Input: part model. Units: mm. Frame: model coordinates. Face numbers are marked on the shaded views. Give positions to 0.01 mm unless a question says otherwise; leave off trailing zeros. Order: outer loops, then holes, each group sorted by start corner. A loop starts at its lowest first (then second) coordinate and runs counter-clockwise, first axis right, second up. Notation, with made-up numbers: (-12.5, 15) - (46.5, 15) arc R15 cw to (46.5, 38) - close; hole circle Ø8 at (-9, 82). An arc over 180 degrees is marked (long way). Use a Markdown table: item, result.
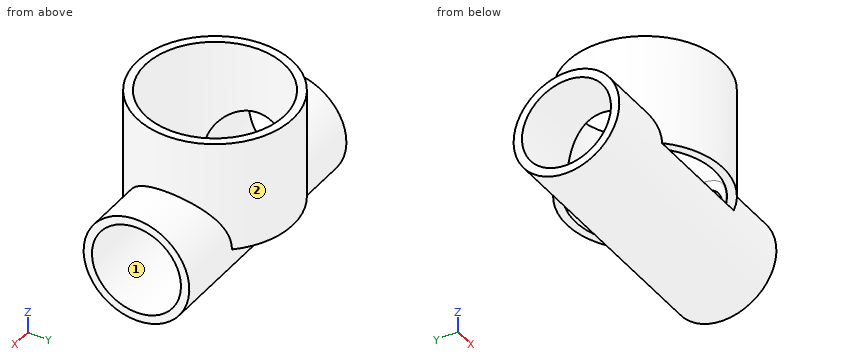
from build123d import *

# Parameters (mm, degrees)
SKETCH_1_R               = 14
SKETCH_1_R_2             = 12.5
EXTRUDE_1_DEPTH          = 20
EXTRUDE_2_DEPTH          = 22.5
EXTRUDE_2_DEPTH_BACK     = 22.5
SKETCH_2_R               = 9.5
SKETCH_2_R_2             = 8
CUT_EXTRUDE_1_DEPTH      = 40.654760284
CUT_EXTRUDE_1_DEPTH_BACK = 20
SKETCH_3_R               = 12.5
CUT_EXTRUDE_2_DEPTH      = 52.195703099
CUT_EXTRUDE_2_DEPTH_BACK = 52.195703099
SKETCH_4_R               = 8


with BuildPart() as part:
    # Sketch 1 → Extrude 1 (new body)
    with BuildSketch(Plane.XY):
        Circle(SKETCH_1_R)
        Circle(SKETCH_1_R_2, mode=Mode.SUBTRACT)
    extrude(amount=EXTRUDE_1_DEPTH)

    # Sketch 2 → Extrude 2 (add, two sides: drawn at the far end of the back side and taken through both)
    with BuildSketch(Plane(origin=(0, 0, 0), x_dir=(0, 0, -1), z_dir=(1, 0, 0)).offset(-EXTRUDE_2_DEPTH_BACK)):
        Circle(SKETCH_2_R)
        Circle(SKETCH_2_R_2, mode=Mode.SUBTRACT)
    extrude(amount=EXTRUDE_2_DEPTH + EXTRUDE_2_DEPTH_BACK)

    # Sketch 3 → Cut-Extrude 1 (cut, two sides: drawn at the far end of the back side and taken through both)
    with BuildSketch(Plane.XY.offset(20).offset(-CUT_EXTRUDE_1_DEPTH_BACK)):
        with Locations(Location((0, 0, 0), (0, 0, 219.7918195))):
            Circle(SKETCH_3_R)
    extrude(amount=CUT_EXTRUDE_1_DEPTH + CUT_EXTRUDE_1_DEPTH_BACK, mode=Mode.SUBTRACT)

    # Sketch 4 → Cut-Extrude 2 (cut, two sides: drawn at the far end of the back side and taken through both)
    with BuildSketch(Plane(origin=(22.5, 0, 0), x_dir=(0, 0, -1), z_dir=(1, 0, 0)).offset(-CUT_EXTRUDE_2_DEPTH_BACK)):
        Circle(SKETCH_4_R)
    extrude(amount=CUT_EXTRUDE_2_DEPTH + CUT_EXTRUDE_2_DEPTH_BACK, mode=Mode.SUBTRACT)


solid = part.part
1. Section query D-D (z = 8.75). Return loops of the section in (x, y).
Response:
| item | result |
|---|---|
| outline | (-22.5, -3.7) - (-13.5, -3.7) arc R14 ccw to (13.5, -3.7) - (22.5, -3.7) - (22.5, 3.7) - (13.5, 3.7) arc R14 ccw to (-13.5, 3.7) - (-22.5, 3.7) - close; hole circle Ø25 at (0, 0) |
2. Pin query (flat end, axial travel): pin 1 (3 mm diameter, centred on x = -7.5, z = 14, fed in from +Y); pin 2 (5 mm diameter, centred on x = 4.5, y = 12.5, fed in from -Z); pin 3 (1.7 mm diameter, centred on x = 4, y = 9, fed in from +Z). Return the tip coordinate at first contact, or that it passes through.
Response:
| item | result |
|---|---|
| pin 1 | stops at y = 12.65 |
| pin 2 | stops at z = 0 |
| pin 3 | stops at z = 0 |
3. Section query C-C (z = -6). Return loops of the section in (x, y).
Response:
| item | result |
|---|---|
| outline | (-22.5, -7.37) - (22.5, -7.37) - (22.5, -5.29) - (-22.5, -5.29) - close; (-22.5, 5.29) - (22.5, 5.29) - (22.5, 7.37) - (-22.5, 7.37) - close |
4. Material intervals for line 1 along X through (y, z) = (0, 15.75); line 2 along Y through (x, z) = (19, 0.25); line 3 along Z through (x, y) = (10, 0), sorted ascending.
Response:
| item | result |
|---|---|
| line 1 | x = -14 to -12.5, 12.5 to 14 |
| line 2 | y = -9.5 to -8, 8 to 9.5 |
| line 3 | z = -9.5 to -8 |
5. Section query B-B (x = -3.5). Return loops of the section in (y, z).
Response:
| item | result |
|---|---|
| outline | (-13.56, 0) - (-12, 0) - (-12, 20) - (-13.56, 20) - close; (-9.5, 0) arc R9.5 ccw to (9.5, 0) - (8, 0) arc R8 cw to (-8, 0) - close; (12, 0) - (13.56, 0) - (13.56, 20) - (12, 20) - close |
6. Mould query, pull axis Y, two halves, no side actions, for the marked faces 1 and 2. Classes: pulls with the +Y half, pulls with the -Y half, needs draft (parallel to the pull), parting line crosses it, or undercut.
Response:
| item | result |
|---|---|
| face 1 | undercut |
| face 2 | parting line crosses it |
7. Section query A-A (y = 0). Return loops of the section in (x, z), then the cut area to 3 significant figures.
Response:
| item | result |
|---|---|
| outline | (-22.5, -9.5) - (22.5, -9.5) - (22.5, -8) - (-22.5, -8) - close; (-22.5, 8) - (-12.5, 8) - (-12.5, 20) - (-14, 20) - (-14, 9.5) - (-22.5, 9.5) - close; (12.5, 8) - (22.5, 8) - (22.5, 9.5) - (14, 9.5) - (14, 20) - (12.5, 20) - close |
| area | 129 mm^2 |
